Geometry: see drawing. Coordinates: mm, zero at the bounding-box minimum. Coordinates: 2 decimals unless noted, no trailing zeros. Write each loop counter-clockwise with the first axis right and the second up, starting at its lowest first coordinate (ties: lowest second). Pieces come first, ordered by that corner, then holes. Notation, with made-up numbers: (-39, 82.5) - (-20, 82.5) arc R21 cw to (-20, 99.5) - close; hole circle Ø1 at (7, -12). An arc over 180 degrees is marked (long way). Use a Markdown table: item, result. Add a question column.
Q1. Section query A-A (x = 21). Return the cut outline in (y, z).
Q2. Section query B-B (y = 36.5). Return the cut outline in (x, z).
Q3. Pin query (flat end, axial travel): P1, Ø1.9, axis at x = 6.5, y = 37.5, coming from the +Z side. Return the tip coordinate at first contact, or that it passes through.
Q4. Section query D-D (z = 0.2). Return the cut outline in (x, y).
Q5. Material intervals for probe 1 along Y at (x, z) = (21, 0.5); probe 2 along X at (y, z) = (22.5, 0.2); probe 3 along X at (y, z) = (8, 0.15) (1 decimal), sorted ascending. Write a range as from..to.
Q6. Section query C-C (y = 23). Return the cut outline in (x, z).
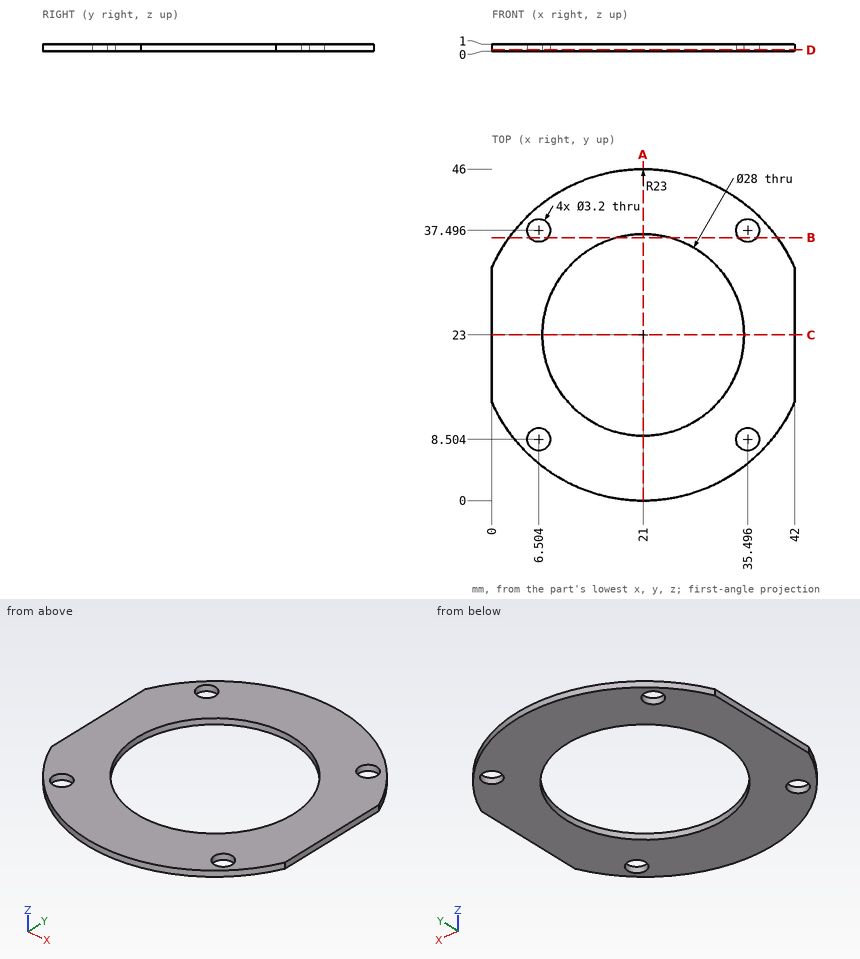
Values follow:
| question | item | result |
|---|---|---|
| 1 | outline | (0, 0) - (9, 0) - (9, 1) - (0, 1) - close; (37, 0) - (46, 0) - (46, 1) - (37, 1) - close |
| 2 | outline | (2.38, 0) - (5.25, 0) - (5.25, 1) - (2.38, 1) - close; (7.76, 0) - (17.29, 0) - (17.29, 1) - (7.76, 1) - close; (24.71, 0) - (34.24, 0) - (34.24, 1) - (24.71, 1) - close; (36.75, 0) - (39.62, 0) - (39.62, 1) - (36.75, 1) - close |
| 3 | P1 | through |
| 4 | outline | (0, 13.62) arc R23 ccw to (42, 13.62) - (42, 32.38) arc R23 ccw to (0, 32.38) - close; hole circle Ø3.2 at (6.5, 8.5); hole circle Ø3.2 at (6.5, 37.5); hole circle Ø28 at (21, 23); hole circle Ø3.2 at (35.5, 8.5); hole circle Ø3.2 at (35.5, 37.5) |
| 5 | probe 1 | 0..9, 37..46 |
| 5 | probe 2 | 0..7.01, 34.99..42 |
| 5 | probe 3 | 3.6..5, 8..34, 37..38.4 |
| 6 | outline | (0, 0) - (7, 0) - (7, 1) - (0, 1) - close; (35, 0) - (42, 0) - (42, 1) - (35, 1) - close |
